Drawing for the job (mm, zero at the part's lowest x, y, z). Coordinates: 2 decimals unless noted, no trailing zeros. Loops run counter-clockwise (first coordinate to the right, second up) from the corner with the lowest first, then second, coordinate; pieces in that order, holes last. Notation, with made-up numbers: (36.25, -36) - (80.25, -36) arc R18 ccw to (80.25, -20) - close; hole circle Ø1 at (-15, 3.5). An arc over 180 degrees is marked (long way). Put each result on its own line as item: value.
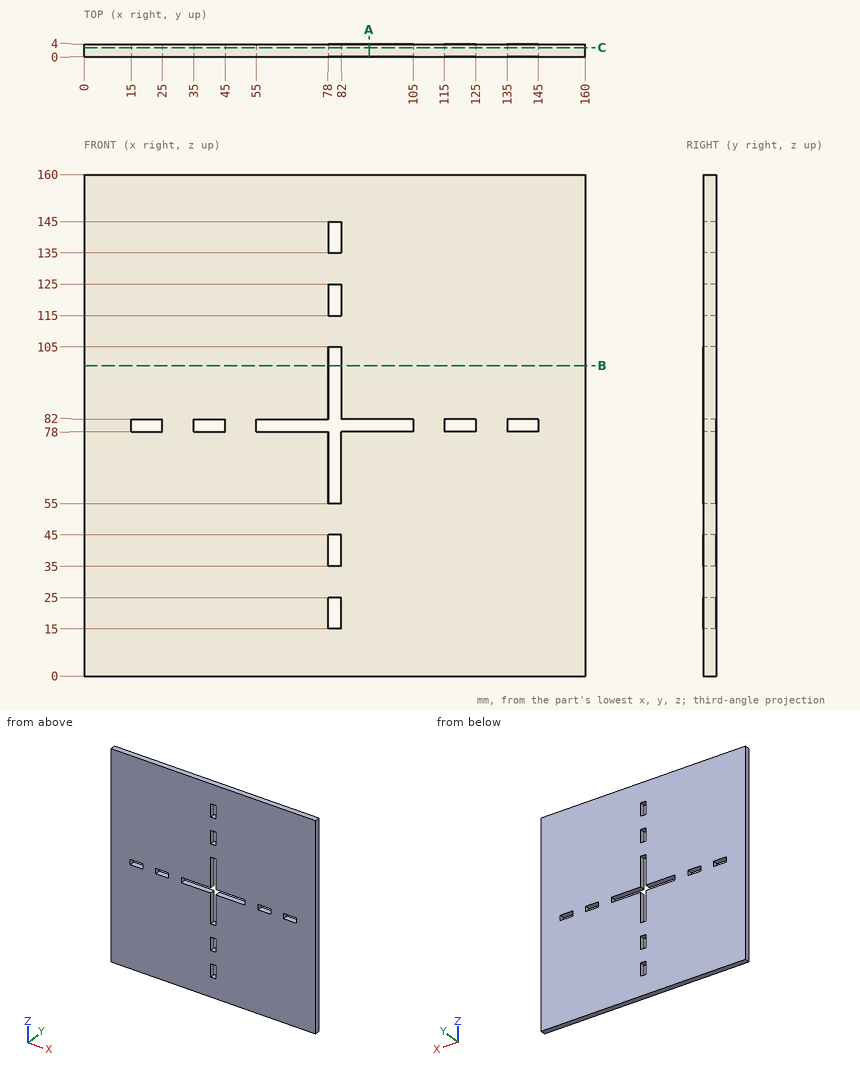
Q1. Pin check, flat tip, straight feed: pin 1 Ø2 at (x, y) = (20, 1.5) entering from -Z. Stop position of the tip, or through.
Determined:
pin 1: z = 0
Q2. Slice it at B-B, the plane z = 99. Give the cut face in (x, y), then the cut area to 3 significant figures.
Determined:
outline: (0, 0) - (78, 0) - (78, 4) - (0, 4) - close; (82, 0) - (160, 0) - (160, 4) - (82, 4) - close
area: 624 mm2
Q3. Wall check: L1, parallel to X at y = 3.4, z = 84; L2, parallel to Z at x = 79.5, y = 1.7. Give the ranges that are in metal, low to high. Write a range as from..to.
Determined:
L1: 0..78, 82..160
L2: 0..15, 25..35, 45..55, 105..115, 125..135, 145..160
Q4. Slice it at C-C, the plane y = 2.85. State how many separate pieces and enclosed holes the cut face has, then the cut area to 3 significant figures.
Determined:
separate pieces: 1
enclosed holes: 9
area: 24,900 mm2
Q5. Slice it at A-A, the plane x = 91. Give the cut face in (y, z), then the cut area to 3 significant figures.
Determined:
outline: (0, 0) - (4, 0) - (4, 78) - (0, 78) - close; (0, 82) - (4, 82) - (4, 160) - (0, 160) - close
area: 624 mm2
